The drawing under review shows one solid part. Ordinate dimensions are in mm from its lowest x, y, z. A direction names the side the tool comes from. Coordinates: 2 decimals unless noted, no trailing zeros. Write each loop counter-clockwise with the first axis right and the second up, starting at its lowest first coordinate (ties: lowest second). Pieces come first, ordered by that corner, then holes.
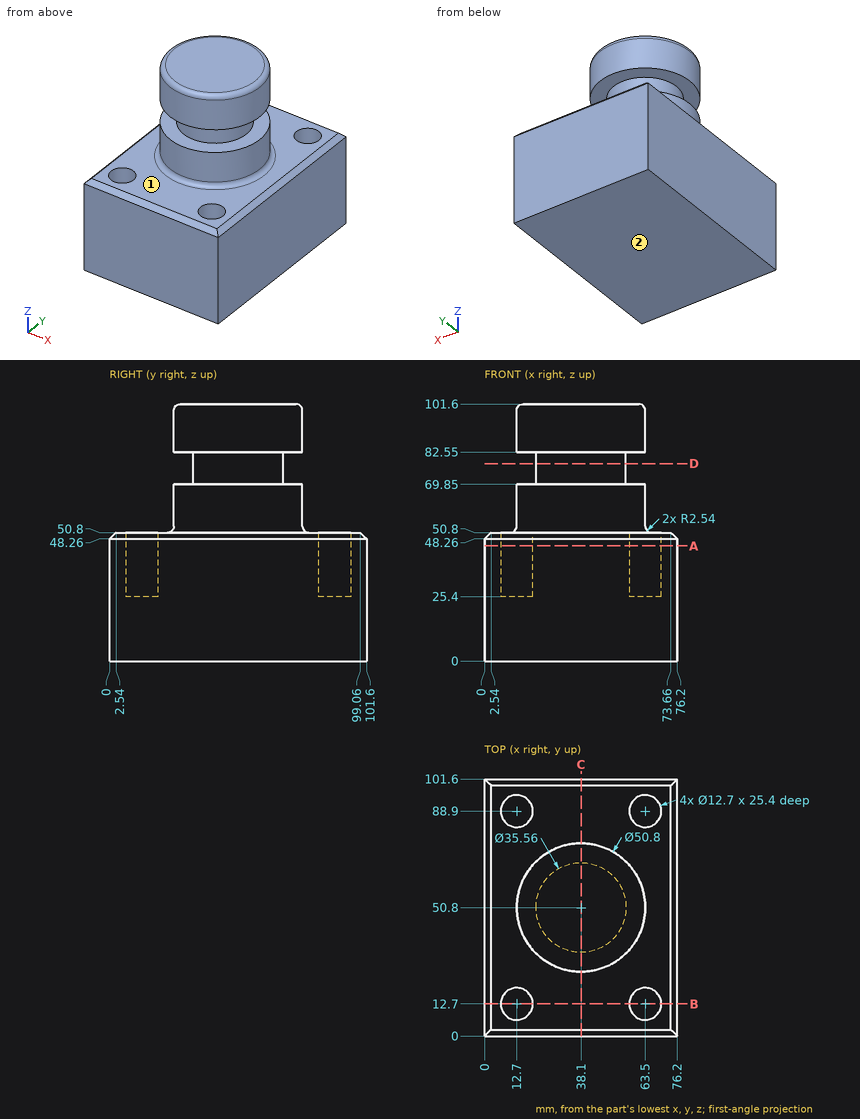
1) Tool access review of the marked faces 1 and 2: name each direction out of +Z, -Z, +X, -X, +Y, -Y from which nothing blocks a thin tool from reaching the whole face with its end or side.
2) Consider section B-B (y = 12.7). Give the boundary of the cut face in (x, z).
3) Consider section D-D (z = 78). Give the boundary of the cut face in (x, y), then the cut area to 3 significant figures.
4) For L1, parallel to Y at x = 63.5, z = 45; L2, parallel to Y at x = 61, z = 40.5; L3, parallel to X at y = 12, z = 34, list the stretches that pass through material, from the lowest coordinate up.
5) Clearance check with flat-ended pins moving along their axes: P1, Ø12, axis at x = 28, z = 72, coming from the -Y side; P2, Ø10, axis at x = 11, y = 14, coming from the +Z side; P3, Ø12, axis at x = 47, y = 19.5, coming from the +Z side; P4, Ø10, axis at x = 12.7, y = 88.9, coming from the -Z side. State where each tip first meets the part, or that it passes through.
6) Consider section A-A (z = 45.5). Give the boundary of the cut face in (x, y), then the cut area to 3 significant figures.
7) Consider section C-C (x = 38.1). Give the boundary of the cut face in (y, z), then the cut area to 3 significant figures.
Results:
1. face 1: +Z
1. face 2: -Z, +X, -X, +Y, -Y
2. outline: (0, 0) - (76.2, 0) - (76.2, 48.26) - (73.66, 50.8) - (69.85, 50.8) - (69.85, 25.4) - (57.15, 25.4) - (57.15, 50.8) - (19.05, 50.8) - (19.05, 25.4) - (6.35, 25.4) - (6.35, 50.8) - (2.54, 50.8) - (0, 48.26) - close
3. outline: circle Ø35.56 at (38.1, 50.8)
3. area: 993 mm2
4. L1: y = 0 to 6.35, 19.05 to 82.55, 95.25 to 101.6
4. L2: y = 0 to 6.86, 18.54 to 83.06, 94.74 to 101.6
4. L3: x = 0 to 6.39, 19.01 to 57.19, 69.81 to 76.2
5. P1: stops at y = 25.8
5. P2: stops at z = 50.8
5. P3: stops at z = 51.22
5. P4: stops at z = 0
6. outline: (0, 0) - (76.2, 0) - (76.2, 101.6) - (0, 101.6) - close; hole circle Ø12.7 at (12.7, 12.7); hole circle Ø12.7 at (12.7, 88.9); hole circle Ø12.7 at (63.5, 12.7); hole circle Ø12.7 at (63.5, 88.9)
6. area: 7,240 mm2
7. outline: (0, 0) - (101.6, 0) - (101.6, 48.26) - (99.06, 50.8) - (78.74, 50.8) arc R2.54 cw to (76.2, 53.34) - (76.2, 69.85) - (68.58, 69.85) - (68.58, 82.55) - (76.2, 82.55) - (76.2, 99.06) arc R2.54 ccw to (73.66, 101.6) - (27.94, 101.6) arc R2.54 ccw to (25.4, 99.06) - (25.4, 82.55) - (33.02, 82.55) - (33.02, 69.85) - (25.4, 69.85) - (25.4, 53.34) arc R2.54 cw to (22.86, 50.8) - (2.54, 50.8) - (0, 48.26) - close
7. area: 7,540 mm2
